The listing builds one solid part. Answer for the finished solid, in the listing's coordinates (mm). Give positions to 0.01 mm unless a question says otherwise; leave off trailing zeros. Loops run counter-clockwise (first coordinate to the right, second up) from the corner with the lowest first, then second, coordinate; pieces in that order, holes last. Notation, with made-up numbers: M 61,-25.5 L 100,-25.5 A19 cw 100,-3.5 Z; hole C 48.5,-8 d10. An arc over 180 degrees is marked long. Return JSON: item names as keys, results as strings.
from build123d import *

# Parameters (mm, degrees)
F0_W     = 4
F0_H     = 5
F1_DEPTH = 4
F2_D     = 3.3
F3_D     = 3.3
F4_W     = 4
F4_H     = 9
F4_W_2   = 10
F4_H_2   = 4
F5_DEPTH = 4
F6_D     = 3.3
F7_R     = 5


with BuildPart() as f1:
    # F0 (on Top) → F1 (new body)
    with BuildSketch(Plane.XY):
        Polygon((18.9080892972, -17.5), (30, -17.5), (30, 17.5), (-30, 17.5), (-30, -17.5), (-18.9080892972, -17.5), (-6.0919107028, -17.5), (6.0919107028, -17.5), align=None)
        with Locations((-26, -11)):
            Rectangle(F0_W, F0_H, mode=Mode.SUBTRACT)
        with Locations((26, -11)):
            Rectangle(F0_W, F0_H, mode=Mode.SUBTRACT)
        with Locations((-26, 11)):
            Rectangle(F0_W, F0_H, mode=Mode.SUBTRACT)
        with Locations((26, 11)):
            Rectangle(F0_W, F0_H, mode=Mode.SUBTRACT)
    extrude(amount=F1_DEPTH)

    # F2 (through all)
    with Locations(Plane(origin=(0, 0, 0), x_dir=(1, 0, 0), z_dir=(0, 0, -1))):
        with Locations((-26, 0), (26, 0)):
            Hole(F2_D / 2)

    # F3 (through all)
    with Locations(Plane(origin=(0, 0, 0), x_dir=(1, 0, 0), z_dir=(0, 0, -1))):
        with Locations((0, 0)):
            Hole(F3_D / 2)

    # F4 (on face) → F5 (join)
    with BuildSketch(Plane.XY.offset(4)):
        Polygon((-36, -77.5), (36, -77.5), (36, 17.5), (36, 35.5), (21, 35.5), (21, 20.5), (0, 20.5), (-21, 20.5), (-21, 35.5), (-36, 35.5), (-36, 17.5), align=None)
        with Locations((-32, -67)):
            Rectangle(F4_W, F4_H, mode=Mode.SUBTRACT)
        with Locations((-21, -73.5)):
            Rectangle(F4_W_2, F4_H_2, mode=Mode.SUBTRACT)
        with Locations((-32, -47)):
            Rectangle(F4_W, F4_H, mode=Mode.SUBTRACT)
        with Locations((-32, -27)):
            Rectangle(F4_W, F4_H, mode=Mode.SUBTRACT)
        with Locations((21, -73.5)):
            Rectangle(F4_W_2, F4_H_2, mode=Mode.SUBTRACT)
        with Locations((32, -67)):
            Rectangle(F4_W, F4_H, mode=Mode.SUBTRACT)
        with Locations((32, -47)):
            Rectangle(F4_W, F4_H, mode=Mode.SUBTRACT)
        with Locations((32, -27)):
            Rectangle(F4_W, F4_H, mode=Mode.SUBTRACT)
        Polygon((-34, 17.5), (-30, 17.5), (30, 17.5), (34, 17.5), (34, 8.5), (30, 8.5), (30, -2.5), (34, -2.5), (34, -11.5), (30, -11.5), (30, -17.5), (-30, -17.5), (-30, -11.5), (-34, -11.5), (-34, -2.5), (-30, -2.5), (-30, 8.5), (-34, 8.5), align=None, mode=Mode.SUBTRACT)
    extrude(amount=-F5_DEPTH)

    # F6 (through all)
    with Locations(Plane.XY.offset(4)):
        with Locations((-32, -37), (32, -37)):
            Hole(F6_D / 2)

    # F7
    f7_edges = [f1.edges().sort_by_distance(p)[0] for p in [
        (-36, -77.5, 2),
        (36, -77.5, 2),
        (-21, 20.5, 2),
        (-21, 35.5, 2),
        (-36, 35.5, 2),
        (21, 35.5, 2),
        (21, 20.5, 2),
        (36, 35.5, 2),
    ]]
    fillet(f7_edges, radius=F7_R)


solid = f1.part
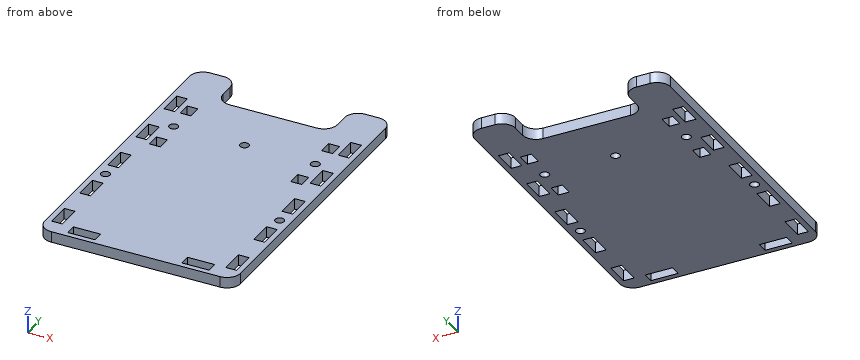
(1) The part is cut by section C-C (z = 1.8). Give the number of separate pieces and of enclosed holes in the cut face, and give its area (3 significant figures).
Values follow:
{"separate pieces": "1", "enclosed holes": "21", "area": "6,920 mm²"}
(2) The part is cut by section D-D (x = 13). Determine the outline of the cut face in (y, z), and give its area (3 significant figures).
Values follow:
{"outline": "M -77.5,0 L 20.5,0 L 20.5,4 L -77.5,4 Z", "area": "392 mm²"}
(3) Given pin 1 (2 mm diameter, centred on x = -32.5, z = 1, fed in from +Y); pin 2 (1.2 mm diameter, centred on x = -5.5, z = 2.5, fed in from +Y); pin 3 (1.2 mm diameter, centred on x = 32.5, z = 1.5, fed in from +Y), each flat-ended and moving along its own axis, determine where each tip first touches the part or whether it passes through.
Values follow:
{"pin 1": "y = 35.47", "pin 2": "y = 20.5", "pin 3": "y = 35.42"}
(4) The part is cut by section B-B (y = 0). Determine the outline of the cut face in (x, z).
Values follow:
{"outline": "M -36,0 L -27.65,0 L -27.65,4 L -36,4 Z; M -24.35,0 L -1.65,0 L -1.65,4 L -24.35,4 Z; M 1.65,0 L 24.35,0 L 24.35,4 L 1.65,4 Z; M 27.65,0 L 36,0 L 36,4 L 27.65,4 Z"}
(5) The part is cut by section A-A (y = -25). Determine the outline of the cut face in (x, z).
Values follow:
{"outline": "M -36,0 L -34,0 L -34,4 L -36,4 Z; M -30,0 L 30,0 L 30,4 L -30,4 Z; M 34,0 L 36,0 L 36,4 L 34,4 Z"}
(6) Straight lines are drawn through the part: line 1 along X through (y, z) = (-45, 1.25); line 2 along Y through (x, z) = (-7, 0.2); line 3 along Y through (x, z) = (-18, 3.5). For each, find the intervals that lie inside material, in ascending order.
Values follow:
{"line 1": "-36 to -34, -30 to 30, 34 to 36", "line 2": "-77.5 to 20.5", "line 3": "-77.5 to -75.5, -71.5 to 20.92"}
